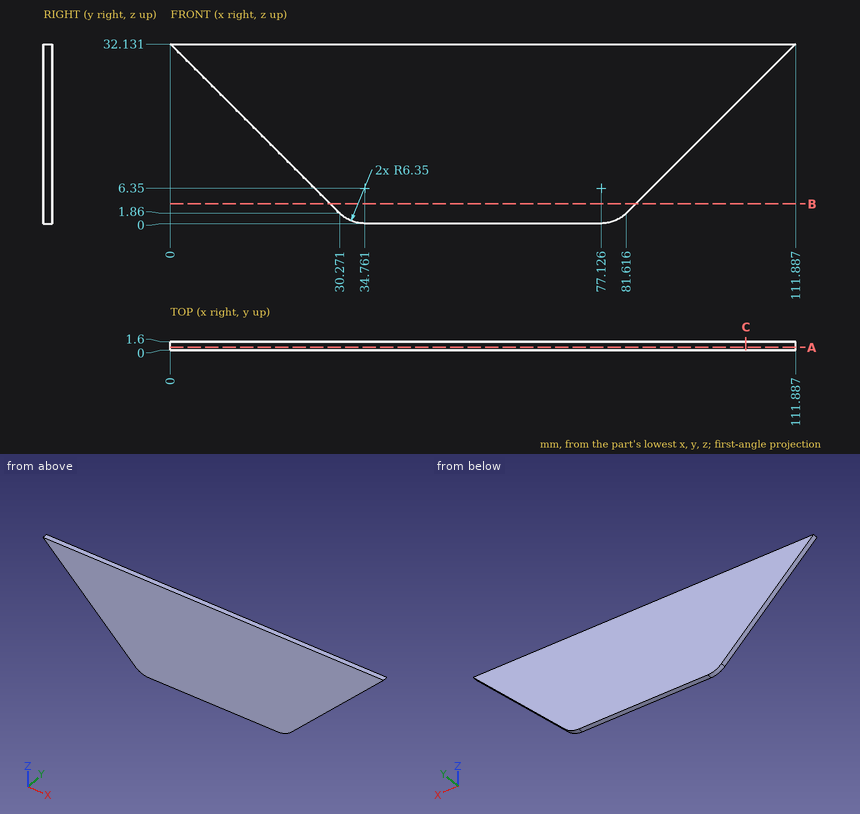
Study the drawing (mm; zero at the part's minimum x, y, z) and answer. Give positions to 0.01 mm unless a question says otherwise; leave off trailing zeros. Write each loop counter-clockwise with the first axis right and the second up, starting at its lowest first coordinate (ties: lowest second). Pieces come first, ordered by that corner, then holes. Notation, with made-up numbers: M 30.5,-17 L 77.5,-17 A24 cw 77.5,-3 Z; hole C -15.75,-8 d8. An arc over 180 degrees is marked long. Put each result on its own line as item: value. Start each with the question number.
1. The part is cut by section B-B, the plane z = 3.5. Give the vertices of the cut face in (x, y).
2. The part is cut by section C-C, the plane x = 103. Give the vertices of the cut face in (y, z).
3. The part is cut by section A-A, the plane y = 0.55. Give the vertices of the cut face in (x, z).
4. Consider line 1 along Z through (x, y) = (84, 1.4) (1 decimal); line 2 along Z through (x, y) = (33, 1.1); line 3 along X through (y, z) = (0.1, 9.5) (1 decimal). Determine where each line is inside the solid, lowest interval first.
Final values:
1. outline: M 28.63,0 L 83.26,0 L 83.26,1.6 L 28.63,1.6 Z
2. outline: M 0,23.24 L 1.6,23.24 L 1.6,32.13 L 0,32.13 Z
3. outline: M 0,32.13 L 30.27,1.86 A6.35 ccw 34.76,0 L 77.13,0 A6.35 ccw 81.62,1.86 L 111.89,32.13 Z
4. line 1: z = 4.2 to 32.1
4. line 2: z = 0.25 to 32.13
4. line 3: x = 22.6 to 89.3
